Study the drawing (mm; zero at the part's minimum x, y, z) and answer. A direction names the side the tool comes from. Give positions to 0.01 mm unless a question says otherwise; leave off trailing zeros. Order: outer loops, then holes, each group sorted by start corner. A loop starts at its lowest first (then second) coordinate and runs counter-clockwise, first axis right, second up. Notation, with made-up numbers: (56.5, -39) - (98.5, -39) arc R19 ccw to (98.5, -34) - close; hole circle Ø7 at (54, -36). An arc over 180 degrees is marked (long way). Return JSON: item names as keys, results as strings.
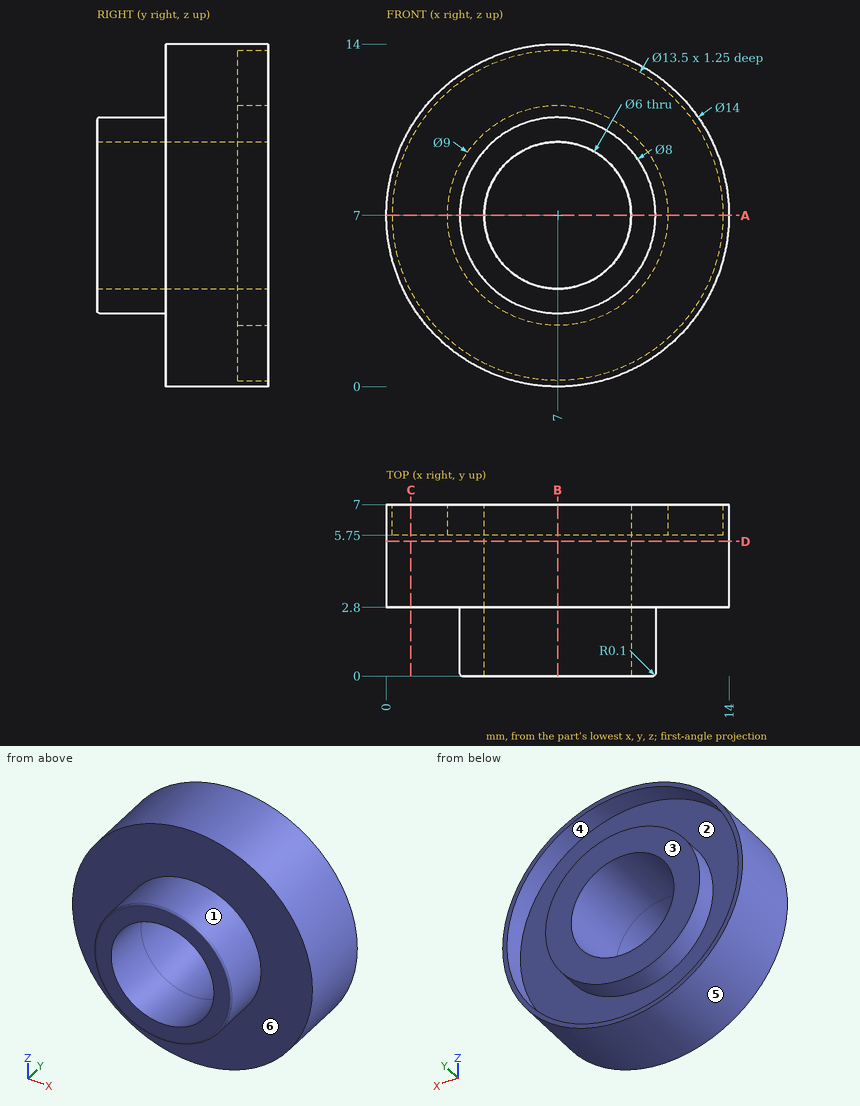
Q1. A cutting plane is placed at A-A (z = 7). Write down the section's boundary in (x, y), and give its area (3 significant figures).
Values:
{"outline": "(0, 2.8) - (3, 2.8) - (3, 0.1) arc R0.1 ccw to (3.1, 0) - (4, 0) - (4, 7) - (2.5, 7) - (2.5, 5.75) - (0.25, 5.75) - (0.25, 7) - (0, 7) - close; (10, 0) - (10.9, 0) arc R0.1 ccw to (11, 0.1) - (11, 2.8) - (14, 2.8) - (14, 7) - (13.75, 7) - (13.75, 5.75) - (11.5, 5.75) - (11.5, 7) - (10, 7) - close", "area": "33.6 mm²"}
Q2. A cutting plane is placed at D-D (y = 5.5). Write down the section's boundary in (x, z), and give its area (3 significant figures).
Values:
{"outline": "circle Ø14 at (7, 7); hole circle Ø6 at (7, 7)", "area": "126 mm²"}
Q3. For the marked faces 1, 2 and 3, determine the directions among +Z, -Z, +X, -X, +Y, -Y from which every point of the face is accessible in a straight line to the end or side of a thin tool.
Values:
{"face 1": "-Y", "face 2": "+Y", "face 3": "+Z, -Z, +X, -X, +Y"}
Q4. Given pin 1 (2 mm diameter, centred on y = 6, z = 10.5, fed in from -X); pin 2 (2 mm diameter, centred on x = 11.5, y = 1.5, fed in from +Z), each flat-ended and moving along its own axis, determine where each tip first touches the part or whether it passes through.
Values:
{"pin 1": "stops at x = 0.46", "pin 2": "stops at z = 8.94"}
Q5. Consider L1, parallel to X at y = 6.75, z = 7; L2, parallel to X at y = 3.75, z = 7. Determine where each line is inside the solid, lowest interval first.
Values:
{"L1": "x = 0 to 0.25, 2.5 to 4, 10 to 11.5, 13.75 to 14", "L2": "x = 0 to 4, 10 to 14"}
Q6. A cutting plane is placed at C-C (x = 1). Write down the section's boundary in (y, z), and give its area (3 significant figures).
Values:
{"outline": "(2.8, 3.39) - (7, 3.39) - (7, 3.91) - (5.75, 3.91) - (5.75, 10.09) - (7, 10.09) - (7, 10.61) - (2.8, 10.61) - close", "area": "22.6 mm²"}
Q7. Determine the mould class of the marked faces 4, 5 and 6 for opening direction X: released by +X, released by -X, zero draft, split by the parting line, or undercut.
Values:
{"face 4": "undercut", "face 5": "split by the parting line", "face 6": "zero draft"}
Q8. A cutting plane is placed at B-B (x = 7). Write down the section's boundary in (y, z), and give its area (3 significant figures).
Values:
{"outline": "(0, 3.1) arc R0.1 ccw to (0.1, 3) - (2.8, 3) - (2.8, 0) - (7, 0) - (7, 0.25) - (5.75, 0.25) - (5.75, 2.5) - (7, 2.5) - (7, 4) - (0, 4) - close; (0, 10) - (7, 10) - (7, 11.5) - (5.75, 11.5) - (5.75, 13.75) - (7, 13.75) - (7, 14) - (2.8, 14) - (2.8, 11) - (0.1, 11) arc R0.1 ccw to (0, 10.9) - close", "area": "33.6 mm²"}
